Could you check a few things on this drawing? It's one solid part, dimensions in mm from its lowest x, y, z. Round coordinates to 2 decimals unless told otherwise and drop trailing zeros. Loops run counter-clockwise (first coordinate to the right, second up) from the corner with the lowest first, then second, coordinate; pieces in that order, holes last.
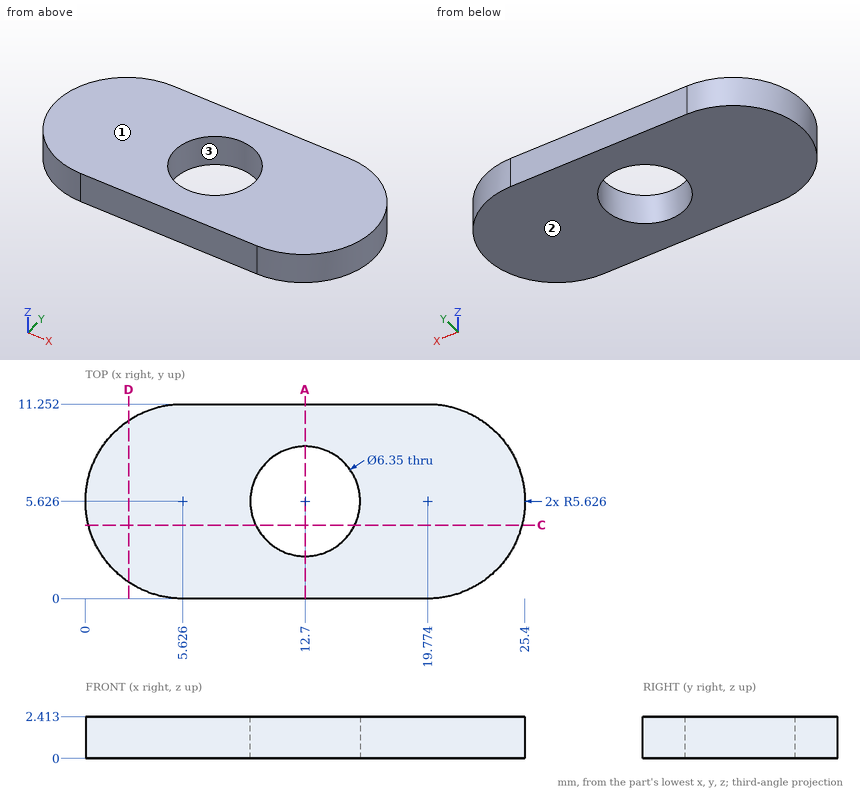
(1) Suppose I cut it at A-A (x = 12.7). Write out the boundary of the cut face in (y, z), then the cut area to 3 significant figures.
(2) Suppose I cut it at D-D (x = 2.5). Write out the boundary of the cut face in (y, z), then the cut area to 3 significant figures.
(3) For pin 1 (1 mm diameter, centred on y = 3, z = 2, fed in from +X), with a flat end and sliding along its axis, tell me the tip position at first contact or that it passes through.
(4) Suppose I cut it at C-C (y = 4.25). Write out the boundary of the cut face in (x, z).
(5) We'd pull the mould along Z, two halves only. Please class the marked faces 1, 2 and 3: released by +Z, released by -Z, zero draft, split by the parting line, or undercut.
(6) If I drill on line 1 (Y direction, x = 12.7, z = 1); line 2 (Y direction, x = 10.5, z = 1.1) (1 decimal); line 3 (X direction, y = 5, z = 1.6) (1 decimal), over which ranges is the centre line in solid material (lowest first)?
Check result:
1. outline: (0, 0) - (2.45, 0) - (2.45, 2.41) - (0, 2.41) - close; (8.8, 0) - (11.25, 0) - (11.25, 2.41) - (8.8, 2.41) - close
1. area: 11.8 mm2
2. outline: (0.95, 0) - (10.3, 0) - (10.3, 2.41) - (0.95, 2.41) - close
2. area: 22.6 mm2
3. pin 1: stops at x = 24.98
4. outline: (0.17, 0) - (9.84, 0) - (9.84, 2.41) - (0.17, 2.41) - close; (15.56, 0) - (25.23, 0) - (25.23, 2.41) - (15.56, 2.41) - close
5. face 1: released by +Z
5. face 2: released by -Z
5. face 3: zero draft
6. line 1: y = 0 to 2.45, 8.8 to 11.25
6. line 2: y = 0 to 3.3, 7.9 to 11.3
6. line 3: x = 0 to 9.6, 15.8 to 25.4
